Autodesk Inventor part; units mm, degrees
ref_plane "YZ Plane" through (0, 0, 0) normal (1, 0, 0) x (0, 1, 0)
ref_plane "XZ Plane" through (0, 0, 0) normal (0, 1, 0) x (-1, 0, 0)
ref_plane "XY Plane" through (0, 0, 0) normal (0, 0, 1) x (1, 0, 0)
sketch "Esquisse1" plane through (0, 0, 0) normal (0, 0, 1) x (1, 0, 0)
  line L0 (-12.8425, 2.6828) -> (-2.685, 7.7657)
  line L1 (2.685, 7.7657) -> (12.8425, 2.6828)
  line L2 (12.8425, -2.6828) -> (2.685, -7.7657)
  line L3 (-2.685, -7.7657) -> (-12.8425, -2.6828)
  arc A0 (2.685, 7.7657) -> (-2.685, 7.7657) centre (0, 2.4) ccw
  arc A1 (-2.685, -7.7657) -> (2.685, -7.7657) centre (0, -2.4) ccw
  arc A2 (-12.8425, 2.6828) -> (-12.8425, -2.6828) centre (-11.5, 0) ccw
  arc A3 (12.8425, -2.6828) -> (12.8425, 2.6828) centre (11.5, 0) ccw
  point P0 (0, 0)
  point P1 (0, 9.1093)
  point P2 (18.2039, 0)
  point P3 (0, -9.1093)
  point P4 (-18.2039, 0)
  dimension "d0" = 6
  dimension "d1" = 3
  dimension "d2" = 29
  dimension "d3" = 16.8
extrude "Extrusion1" add sketch "Esquisse1" along normal blind 0.9
sketch "Esquisse2" plane through (0, 0, 0.9) normal (0, 0, 1) x (1, 0, 0)
  point P0 (0, 0)
  point P1 (0, 0)
hole "Perçage D6" at (0, 0, 0.9) direction (0, 0, -1) diameter 6 end through all
sketch "Esquisse3" plane through (0, 0, 0.9) normal (0, 0, 1) x (1, 0, 0)
  point P0 (0, 0)
  point P1 (-10, 0)
  point P2 (10, 0)
  dimension "d13" = 20
  dimension "d21" = 10
hole "Perçage D3.15" at (-10, 0, 0.9) at (10, 0, 0.9) direction (0, 0, -1) diameter 3.15 end through all
properties part number "Maintient roulement" material "Aluminium"
Source: CAD feature listing. Evaluate the final solid. Frame: model axes, mm. Give positions to 0.01 mm unless a question says otherwise; leave off trailing zeros. Loops run counter-clockwise (first coordinate to the right, second up) from the corner with the lowest first, then second, coordinate; pieces in that order, holes last. Notation, with made-up numbers: M 41,82.25 L 52,82.25 A24 ccw 52,95.25 Z; hole C 53.5,18 d1. An arc over 180 degrees is marked long. Put each result on its own line as item: value.
Q1. Mould query, pull axis Y, two halves, no side actions, for faces 1 (the cylindrical face through (-8.462, 0.341, 0.444)), 2 (the flat face through (-3.4, 0.1, 0.9)), 3 (the cylindrical face through (0, -8.4, 0.4)), 4 (the flat face through (-7.83, 5.19, 0.44)). Classes: released by +Y, released by -Y, zero draft, split by the parting line, or undercut.
Response values:
face 1: undercut
face 2: zero draft
face 3: released by -Y
face 4: released by +Y
Q2. Section A-A (x = 0). Return the cut outline in (y, z), and give its area (3 significant figures).
Response values:
outline: M -8.4,0 L -3,0 L -3,0.9 L -8.4,0.9 Z; M 3,0 L 8.4,0 L 8.4,0.9 L 3,0.9 Z
area: 9.72 mm²
Q3. Section C-C (z = 0.2). Count the separate pieces of the cut face and the enclosed holes in it, and give its area (3 significant figures).
Response values:
separate pieces: 1
enclosed holes: 3
area: 269 mm²
Q4. Section D-D (x = 5.5). Return the cut outline in (y, z), and give its area (3 significant figures).
Response values:
outline: M -6.36,0 L 6.36,0 L 6.36,0.9 L -6.36,0.9 Z
area: 11.4 mm²
Q5. Section B-B (y = 2). Return the cut outline in (x, z), and give its area (3 significant figures).
Response values:
outline: M -13.74,0 L -2.24,0 L -2.24,0.9 L -13.74,0.9 Z; M 2.24,0 L 13.74,0 L 13.74,0.9 L 2.24,0.9 Z
area: 20.7 mm²
Q6. Line query: probe 1 along Y at (x, z) = (0, 0.65); probe 2 along X at (y, z) = (1.25, 0.65); probe 3 along Y at (x, z) = (-10, 0.25) (3 decimals). Output: solid intervals per line, ascending. Write a range as [from, to].
Response values:
probe 1: y = [-8.4, -3], [3, 8.4]
probe 2: x = [-14.23, -10.96], [-9.04, -2.73], [2.73, 9.04], [10.96, 14.23]
probe 3: y = [-4.105, -1.575], [1.575, 4.105]
